Autodesk Inventor part; units mm, degrees
ref_plane "Right" through (0, 0, 0) normal (1, 0, 0) x (0, 1, 0)
ref_plane "Top" through (0, 0, 0) normal (0, 1, 0) x (-1, 0, 0)
ref_plane "Front" through (0, 0, 0) normal (0, 0, 1) x (1, 0, 0)
sketch "Sketch1" plane through (0, 0, 0) normal (1, 0, 0) x (0, 1, 0)
  line L0 (-40, 15) -> (40, 15)
  line L1 (40, 15) -> (40, -15)
  line L2 (40, -15) -> (-40, -15)
  line L3 (-40, -15) -> (-40, 15)
  line L4 (-40, 15) -> (40, -15) construction
  line L5 (40, 15) -> (-40, -15) construction
  point P0 (0, 0)
  dimension "d0" = 30
  dimension "d1" = 80
extrude "Extrusion1" add sketch "Sketch1" along normal mid plane 140.5
sketch "Sketch2" plane through (-70.25, -40, 15) normal (0, 0, 1) x (1, 0, 0)
  line L0 (140.5, 80) -> (0, 80) construction
  line L1 (0, 0) -> (0, 80) construction
  line L2 (0, 80) -> (0, 58.5)
  line L3 (0, 58.5) -> (34.25, 80)
  line L4 (34.25, 80) -> (0, 80)
  line L5 (0, 21.5) -> (0, 0)
  line L6 (0, 0) -> (34.25, 0)
  line L7 (34.25, 0) -> (0, 21.5)
  line L8 (140.5, 80) -> (140.5, 0) construction
  point P0 (70.25, 40)
  dimension "d4" = 37
  dimension "d6" = 147.882
  dimension "d38" = 106.25
extrude "Extrusion2" cut sketch "Sketch2" against normal through all
sketch "Sketch3" plane through (70.25, -40, 15) normal (0, 0, 1) x (1, 0, 0)
  line L0 (0, 80) -> (0, 0) construction
  line L1 (-140.5, 21.5) -> (-140.5, 58.5) construction
  line L2 (-140.5, 57.1) -> (0, 57.1)
  line L3 (0, 57.1) -> (0, 22.9)
  line L4 (0, 22.9) -> (-140.5, 22.9)
  line L5 (-140.5, 22.9) -> (-140.5, 57.1)
  point P0 (-70.25, 40)
  point P1 (-140.5, 40)
  dimension "d9" = 34.2
extrude "Extrusion3" cut sketch "Sketch3" against normal blind 2
sketch "Sketch4" plane through (-36, 40, 15) normal (0, 0, 1) x (1, 0, 0)
  line L0 (106.25, -57.1) -> (-34.25, -57.1) construction
  line L1 (-34.25, -58.5) -> (-34.25, -57.1) construction
  line L2 (-34.25, -58.5) -> (0, -80) construction
  line L3 (0, -80) -> (106.25, -80) construction
  line L4 (106.25, -57.1) -> (106.25, -80) construction
  line L5 (-34.25, -22.9) -> (106.25, -22.9) construction
  line L6 (-34.25, -57.1) -> (-34.25, -22.9) construction
  line L7 (106.25, -57.1) -> (-34.25, -57.1) construction
  line L8 (106.25, -22.9) -> (106.25, -57.1) construction
  line L9 (106.25, -22) -> (80.25, -22)
  line L10 (80.25, -22) -> (80.25, -58)
  line L11 (80.25, -58) -> (106.25, -58)
  line L12 (106.25, -58) -> (106.25, -22)
  line L13 (85.375, -21.875) -> (85.375, -58.125) construction
  line L14 (90.5, -21.875) -> (90.5, -58.125)
  line L15 (80.25, -58.125) -> (80.25, -21.875)
  arc A0 (90.5, -21.875) -> (80.25, -21.875) centre (85.375, -21.875) ccw
  arc A1 (80.25, -58.125) -> (90.5, -58.125) centre (85.375, -58.125) ccw
  point P0 (36, -40)
  point P1 (106.25, -40)
  point P2 (85.375, -40)
  point P3 (80.25, -40)
  dimension "d12" = 36
  dimension "d13" = 26
  dimension "d14" = 46.5
  dimension "d15" = 15.75
extrude "Extrusion4" cut sketch "Sketch4" against normal blind 9.5
sketch "Sketch5" plane through (70.25, -40, 13) normal (0, 0, 1) x (1, 0, 0)
  line L0 (-26, 22.9) -> (-26, 57.1) construction
  line L1 (-15.75, 58) -> (0, 58) construction
  line L2 (-15.75, 58.125) -> (-15.75, 58) construction
  arc A0 (-15.75, 58.125) -> (-26, 58.125) centre (-20.875, 58.125) ccw construction
  line L3 (-26, 21.875) -> (-26, 58.125) construction
  arc A1 (-26, 21.875) -> (-15.75, 21.875) centre (-20.875, 21.875) ccw construction
  line L4 (-15.75, 22) -> (-15.75, 21.875) construction
  line L5 (0, 22) -> (-15.75, 22) construction
  line L6 (0, 58) -> (0, 22) construction
  line L7 (-90.5, 40) -> (-50.5, 40)
  circle A2 centre (-90.5, 40) radius 4.25
  circle A3 centre (-50.5, 40) radius 4.25
  point P0 (-70.25, 40)
  dimension "d18" = 8.5
  dimension "d19" = 48.5
  dimension "d20" = 20.25
  dimension "d23" = 50.5
  dimension "d24" = 40
hole "Hole1" at (-20.25, 0, 13) at (19.75, 0, 13) direction (0, 0, -1) diameter 8.509 end through all
sketch "Sketch6" plane through (70.25, 0, 0) normal (1, 0, 0) x (0, 0, -1)
  line L0 (15, -40) -> (15, 40) construction
  line L1 (15, 40) -> (-15, 40) construction
  line L2 (15, -40) -> (-6.4359, 40)
  line L3 (-6.4359, 40) -> (15, 40)
  line L4 (15, 40) -> (15, -40)
  point P0 (0, 0)
  dimension "d32" = 15
extrude "Extrusion5" cut sketch "Sketch6" against normal through all
move faces "Move1" translate (2.5, 0, 0) faces at (70.25, -13.3333, -1.3333)
equation "\"BendRadius\" = Thickness"
equation "\"BendReliefWidth\" = 0.5 * Thickness"
equation "\"BendReliefDepth\" = 0.5 * Thickness"
equation "\"CornerReliefSize\" = 4 * Thickness"
equation "\"MinimumRemnant\" = 2 * Thickness"
equation "\"TransitionRadius\" = BendRadius"
equation "\"JacobiRadiusSize\" = BendRadius"
properties part number "DHC-1500-FF-02-003-CAST" material "A36"
Model file for the job. Use its own axes, mm. A direction names the side the tool comes from. Round coordinates to 2 decimals unless told otherwise and drop trailing zeros. Write each loop counter-clockwise with the first axis right and the second up, starting at its lowest first coordinate (ties: lowest second). Pieces come first, ordered by that corner, then holes. Notation, with made-up numbers: M 5,61.25 L 12,61.25 A35 ccw 12,93.25 Z; hole C 6,-11 d2. An arc over 180 degrees is marked long. Put each result on its own line as item: value.
Item 1: Cut at B-B (y = 0). List the corners of the cut face in (x, z), and give its area (3 significant figures).
Responses:
outline: M -70.25,-4.28 L -24.5,-4.28 L -24.5,13 L -70.25,13 Z; M -16,-4.28 L 15.5,-4.28 L 15.5,13 L -16,13 Z; M 24,-4.28 L 72.75,-4.28 L 72.75,5.5 L 44.25,5.5 L 44.25,13 L 24,13 Z
area: 1,960 mm²
Item 2: Mould opens along X. For faces 4 (the flat face through (-70.25, 0, 3)), 5 (the cylindrical face through (49.49, 23.25, 10.32)), 6 (the flat face through (64, 18, 10)), 7 (the cylindrical face through (49.26, -23.25, 10.32)) say: +X half, -X half, draft (parallel to the pull), parting line (faces both ways), or undercut.
Responses:
face 4: -X half
face 5: undercut
face 6: draft
face 7: undercut
Item 3: Tool access for faces 1 (the flat face through (-14, 0, 13)), 2 (the flat face through (72.75, -9, 4)), 3 (the flat face through (63, -18, 10)): list every direction of +Z, -Z, +X, -X, +Y, -Y with a clear straight run to the whole face (end or side of a thin tool).
Responses:
face 1: +Z, +X, -X
face 2: +Z, -Z, +X, +Y, -Y
face 3: +Z, +X
Item 4: Cut at A-A (z = 11). State how many separate pieces and enclosed holes the cut face has, and give its area (3 significant figures).
Responses:
separate pieces: 1
enclosed holes: 2
area: 9,480 mm²
Item 5: Cut at C-C (x = 19.75). List the corners of the cut face in (y, z).
Responses:
outline: M -40,-15 L -4.25,-5.42 L -4.25,13 L -17.1,13 L -17.1,15 L -40,15 Z; M 4.25,-3.14 L 40,6.44 L 40,15 L 17.1,15 L 17.1,13 L 4.25,13 Z
Item 6: Probe L1, parallel to X at y = 0, z = 1.25; L2, parallel to X at y = 0, z = 8.25; L3, parallel to Y at x = -45, z = 13.5. List the from-to ranges inside material, lowest first. Write a range as from..to.
Responses:
L1: -70.25..-24.5, -16..15.5, 24..72.75
L2: -70.25..-24.5, -16..15.5, 24..44.25
L3: -34.35..-17.1, 17.1..34.35
Item 7: Flat gauge pins, fed straight in: P1, Ø0.6, axis at x = -39, z = 14.5, coming from the -Y side; P2, Ø5, axis at y = -2, z = 9.5, coming from the +X side; P3, Ø7.5, axis at x = 19.75, y = 0, coming from the -Z side; P4, Ø8, axis at x = -38, y = -11.5, coming from the -Z side. Where does each tip first touch, or does it go through?
Responses:
P1: y = -38.31
P2: x = 44.25
P3: through
P4: z = -8.44
Item 8: Cut at D-D (x = -48). List the corners of the cut face in (y, z), and give its area (3 significant figures).
Responses:
outline: M -32.47,-12.98 L 32.47,4.42 L 32.47,15 L 17.1,15 L 17.1,13 L -17.1,13 L -17.1,15 L -32.47,15 Z
area: 1,180 mm²
